Here's how the part is built. I have some questions about the finished solid (model axes, mm). Face numbers are marked on the shaded views. A direction names the side the tool comes from. Coordinates: 2 decimals unless noted, no trailing zeros. Write each loop counter-clockwise with the first axis right and the second up, starting at its lowest first coordinate (ties: lowest second). Pieces come first, ordered by that corner, then holes. Notation, with made-up numbers: (21.5, 1.25) -> (75.5, 1.25) arc R21 cw to (75.5, 31.25) -> close; hole circle Ø11 at (78, -5). An arc over 180 degrees is marked (long way). Put each result on its own line as item: value. Start each with the question number.
Item 1: I want a section at B-B, the plane x = 54. List the corners of the cut face in (y, z) for me.
Item 2: I want a section at C-C, the plane y = 17. List the corners of the cut face in (x, z) for me, then the cut area to 3 significant figures.
Item 3: I want a section at D-D, the plane z = 14. List the corners of the cut face in (x, y) for me.
Item 4: I want a section at A-A, the plane x = 156. List the corners of the cut face in (y, z) for me.
Item 5: On a 3-axis mill with a long thin cutter (end or side, diameter ignored), from which of +Z, -Z, +X, -X, +Y, -Y can I reach the whole of each face in a straight line? I mean the marked faces 5 and 6. Say none if no direction works.
Item 6: If we mould it in two halves opening along Y, with no side actions, what happens to the marked faces 1, 2, 3 and 4? For each: released by +Y, released by -Y, zero draft, split by the parting line, or undercut.
Item 7: For pin 1 (4 mm diameter, centred on y = 28.5, z = 8, fed in from -X); pin 2 (8 mm diameter, centred on y = 9.5, z = 9.5, fed in from +X); pin 3 (3.5 mm diameter, centred on x = -12, z = 6.5, fed in from -Y), each with a flat end and sliding along its axis, tell me the tip position at first contact or that it passes through.
Item 8: I need wall thicknesses on line 1 (Y direction, x = 6, z = 1.25); line 2 (Y direction, x = -2.35, z = 10); line 3 (Z direction, x = -5, y = -10). Which ranges of each line are inside material? Lowest first, please. Write a range as [from, to].
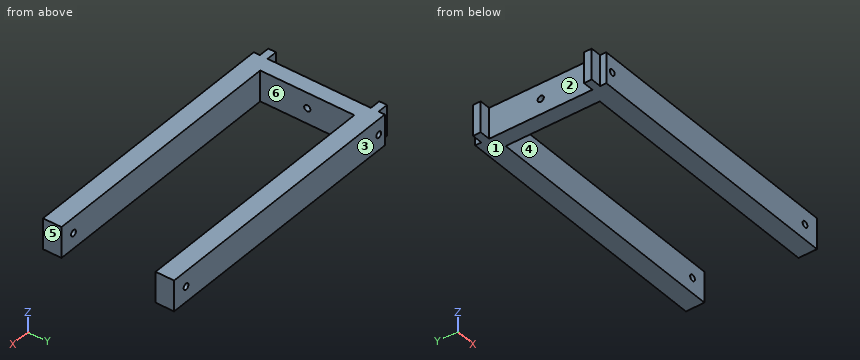
from build123d import *

# Parameters (mm, degrees)
PAD_DEPTH       = 20
SKETCH004_R     = 2
POCKET002_DEPTH = 176.001
SKETCH005_R     = 2
POCKET003_DEPTH = 85.001


with BuildPart() as part:
    # Sketch → Pad (new body)
    with BuildSketch(Plane.XY):
        Polygon((-10, -42.5), (166, -42.5), (166, -30.5), (0, -30.5), (0, 30.5), (166, 30.5), (166, 42.5), (-10, 42.5), (-10, 38.5), (-17, 38.5), (-17, 33.5), (-10, 33.5), (-10, -33.5), (-17, -33.5), (-17, -38.5), (-10, -38.5), align=None)
    extrude(amount=PAD_DEPTH)

    # Sketch004 → Pocket002 (cut, through all)
    with BuildSketch(Plane(origin=(-10, 0, 0), x_dir=(0, -1, 0), z_dir=(-1, 0, 0))):
        with Locations((0, 10)):
            Circle(SKETCH004_R)
    extrude(amount=-POCKET002_DEPTH, mode=Mode.SUBTRACT)

    # Sketch005 → Pocket003 (cut, through all)
    with BuildSketch(Plane.XZ.offset(42.5)):
        with Locations((-5, 10)):
            Circle(SKETCH005_R)
        with Locations((156, 10)):
            Circle(SKETCH005_R)
    extrude(amount=-POCKET003_DEPTH, mode=Mode.SUBTRACT)


solid = part.part
Calculated:
1. outline: (-42.5, 0) -> (-30.5, 0) -> (-30.5, 20) -> (-42.5, 20) -> close; (30.5, 0) -> (42.5, 0) -> (42.5, 20) -> (30.5, 20) -> close
2. outline: (-10, 0) -> (0, 0) -> (0, 20) -> (-10, 20) -> close; hole circle Ø4 at (-5, 10)
2. area: 187 mm2
3. outline: (-17, -38.5) -> (-10, -38.5) -> (-10, -42.5) -> (166, -42.5) -> (166, -30.5) -> (0, -30.5) -> (0, 30.5) -> (166, 30.5) -> (166, 42.5) -> (-10, 42.5) -> (-10, 38.5) -> (-17, 38.5) -> (-17, 33.5) -> (-10, 33.5) -> (-10, -33.5) -> (-17, -33.5) -> close
4. outline: (-42.5, 0) -> (-30.5, 0) -> (-30.5, 8) -> (-42.5, 8) -> close; (-42.5, 12) -> (-30.5, 12) -> (-30.5, 20) -> (-42.5, 20) -> close; (30.5, 0) -> (42.5, 0) -> (42.5, 8) -> (30.5, 8) -> close; (30.5, 12) -> (42.5, 12) -> (42.5, 20) -> (30.5, 20) -> close
5. face 5: +Z, -Z, +X, +Y, -Y
5. face 6: +Z, -Z, +X
6. face 1: zero draft
6. face 2: undercut
6. face 3: released by +Y
6. face 4: undercut
7. pin 1: stops at x = -10
7. pin 2: stops at x = 0
7. pin 3: stops at y = -38.5
8. line 1: y = [-42.5, -30.5], [30.5, 42.5]
8. line 2: y = [-42.5, -2], [2, 42.5]
8. line 3: z = [0, 8], [12, 20]
